Geometry: final body of the model. Coordinates: model frame, mm. Coordinates: 2 decimals unless noted, no trailing zeros. Order: outer loops, then holes, each group sorted by start corner. A loop starts at its lowest first (then second) coordinate and runs counter-clockwise, first axis right, second up. Notation, with made-up numbers: M -15,-22.75 L 17,-22.75 A16 ccw 17,-8.75 Z; hole C 1,68 d5. An arc over 180 degrees is marked long. Write item = value, one per line.
from build123d import *

# Parameters (mm, degrees)
F0_W        = 63.7673679739
F0_H        = 29.4773685746
F1_DEPTH    = 93.472
F2_R        = 5.08
F3_T1_DEPTH = 113.792
F3_T3_DEPTH = 54.8773685746
F4_T1_DEPTH = 79.007367974


# Not quite as in the source:
# - a fillet or chamfer that OpenCascade refuses, or shapes differently, is made with other operations: its cross-section is extruded or revolved along the edge and cut away or added
# - the program builds the solid bodies; features that only make, move or delete a surface that nothing else refers to are left out


with BuildPart() as f1:
    # F0 (on Front) → F1 (new body)
    with BuildSketch(Plane.XZ):
        with Locations((-3.0078953132, 7.5197371189)):
            Rectangle(F0_W, F0_H)
    extrude(amount=F1_DEPTH)

    # F2
    f2_edges = [f1.edges().sort_by_distance(p)[0] for p in [
        (-3.007895, -93.472, 22.258421),
        (-34.891579, -93.472, 7.519737),
        (-3.007895, -93.472, -7.218947),
        (28.875789, -93.472, 7.519737),
        (28.875789, -46.736, -7.218947),
        (28.875789, -46.736, 22.258421),
        (28.875789, 0, 7.519737),
    ]]
    fillet(f2_edges, radius=F2_R)

    # F3: fillet of radius 5.08 on 4 edges, made by hand

    # F3_s2 → F3_t1 (cut)
    with BuildSketch(Plane.XZ.offset(-12.7)):
        with BuildLine():
            ThreePointArc((-29.8115793002, 22.2584214061), (-33.4036817486, 20.7705238546), (-34.8915793002, 17.1784214061))
            Line((-34.8915793002, 17.1784214061), (-34.8915793002, 22.2584214061))
            Line((-34.8915793002, 22.2584214061), (-29.8115793002, 22.2584214061))
        make_face()
        with BuildLine():
            ThreePointArc((-34.8915793002, -2.1389471684), (-33.4036817486, -5.7310496169), (-29.8115793002, -7.2189471684))
            Line((-29.8115793002, -7.2189471684), (-34.8915793002, -7.2189471684))
            Line((-34.8915793002, -7.2189471684), (-34.8915793002, -2.1389471684))
        make_face()
    extrude(amount=F3_T1_DEPTH, mode=Mode.SUBTRACT)

    # F3_s4 → F3_t3 (cut)
    with BuildSketch(Plane.XY.offset(-19.9189471684)):
        with BuildLine():
            ThreePointArc((-34.8915793002, -5.08), (-33.4036817486, -1.4878975516), (-29.8115793002, 0))
            Line((-29.8115793002, 0), (-34.8915793002, 0))
            Line((-34.8915793002, 0), (-34.8915793002, -5.08))
        make_face()
    extrude(amount=F3_T3_DEPTH, mode=Mode.SUBTRACT)

    # F4: fillet of radius 5.08 on 4 edges, made by hand

    # F4_s2 → F4_t1 (cut)
    with BuildSketch(Plane.YZ.offset(-42.5115793002)):
        with BuildLine():
            ThreePointArc((0, -2.1389471684), (-1.4878975516, -5.7310496169), (-5.08, -7.2189471684))
            Line((-5.08, -7.2189471684), (0, -7.2189471684))
            Line((0, -7.2189471684), (0, -2.1389471684))
        make_face()
        with BuildLine():
            ThreePointArc((-5.08, 22.2584214061), (-1.4878975516, 20.7705238546), (0, 17.1784214061))
            Line((0, 17.1784214061), (0, 22.2584214061))
            Line((0, 22.2584214061), (-5.08, 22.2584214061))
        make_face()
    extrude(amount=F4_T1_DEPTH, mode=Mode.SUBTRACT)


solid = f1.part
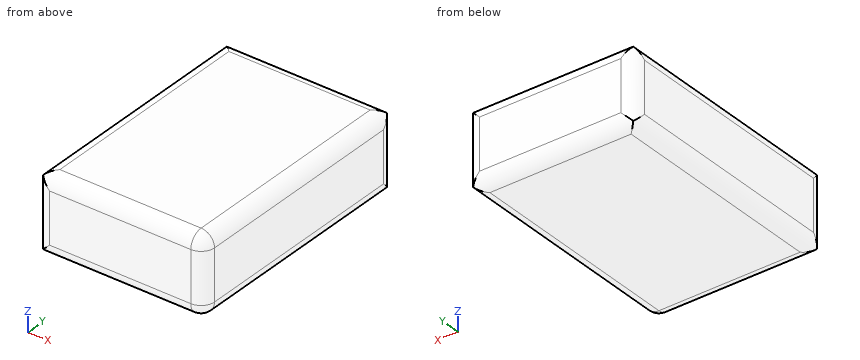
1) Section B-B, the plane z = -3.75. Return loops of the section in (x, y), and give its area (3 significant figures).
Numbers:
outline = M -34.63,-90 A5.08 ccw -31.42,-93.21 L 23.8,-93.21 A4.82 ccw 28.61,-88.39 L 28.61,-3.47 A5.08 ccw 25.41,-0.26 L -31.42,-0.26 A5.08 ccw -34.63,-3.47 Z
area = 5,860 mm²
2) Section A-A, the plane z = 19.25. Return loops of the section in (x, y).
Numbers:
outline = M -34.45,-90.46 A5.08 ccw -31.88,-93.03 L 23.8,-93.03 A4.64 ccw 28.43,-88.39 L 28.43,-3.01 A5.08 ccw 25.87,-0.44 L -31.88,-0.44 A5.08 ccw -34.45,-3.01 Z
3) Line query: L1, parallel to X at y = -34, z = 20.75; L2, parallel to Z at x = 24, y = -22; L3, parallel to Y at x = -30, z = 17.25. Output: solid intervals per line, ascending.
Numbers:
L1 = -33.42 to 27.41
L2 = -7.21 to 22.25
L3 = -93.47 to 0
4) Pin query (flat end, axial travel): pin 1 (8 mm diameter, centred on x = -26.5, z = 18.5, fed in from +Y). Return the tip coordinate at first contact, or that it passes through.
Numbers:
pin_1 = 0
